Answer from the drawing. Dimensions are ordinates in mm from the lowest x, y and z of the part. Give positions to 0.01 mm unless a question says otherwise; leave off trailing zeros. Order: outer loops, then holes, each group sorted by start corner. A loop starts at its lowest first (then second) coordinate and runs counter-clockwise, first axis right, second up.
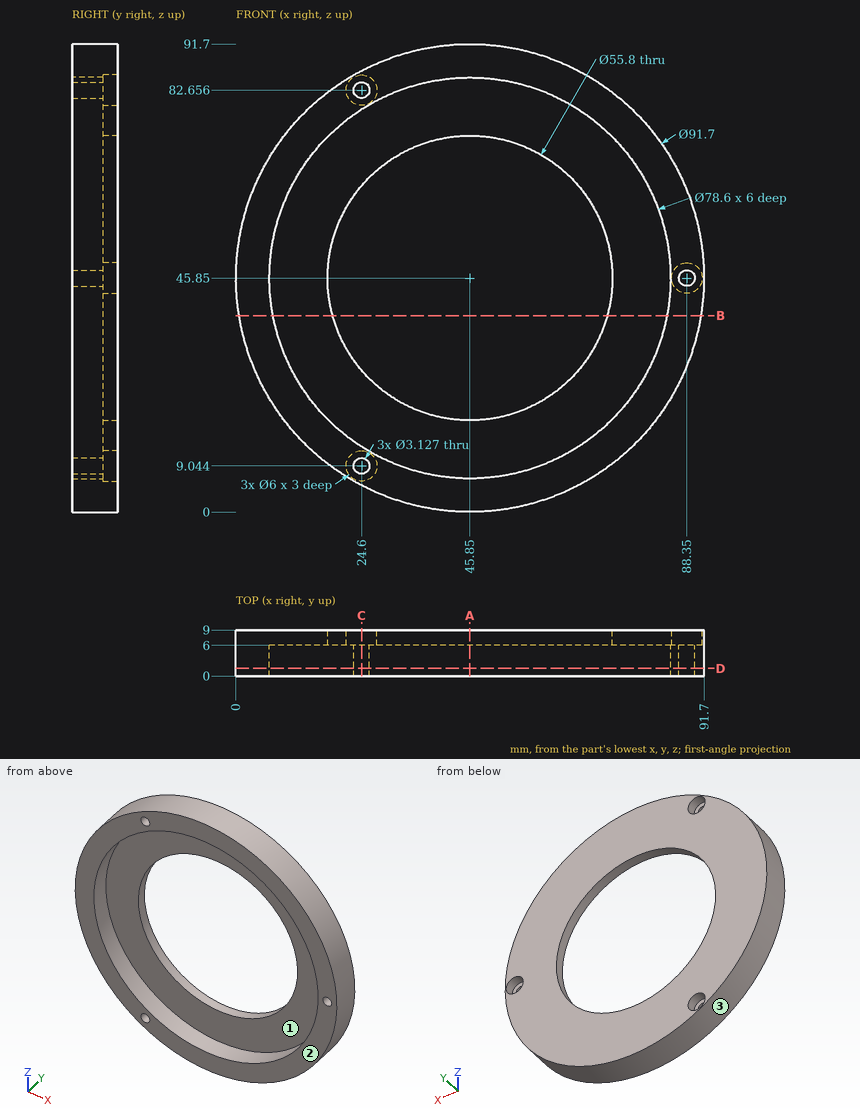
1) For a pull along Z with two mould halves and no side action, classify the marked faces 1, 2 and 3 as released by +Z, released by -Z, zero draft, split by the parting line, or undercut.
Final values:
face 1: undercut
face 2: zero draft
face 3: split by the parting line
2) The part is cut by section D-D on y = 1.5. Determine the outline of the cut face in (x, z).
Final values:
outline: circle Ø91.7 at (45.85, 45.85); hole circle Ø78.6 at (45.85, 45.85); hole circle Ø3.13 at (24.6, 9.04); hole circle Ø3.13 at (24.6, 82.66); hole circle Ø3.13 at (88.35, 45.85)
3) Given pin 1 (5 mm diameter, centred on x = 35.5, z = 18.5, fed in from -Y); pin 2 (4 mm diameter, centred on x = 40, y = 5.5, fed in from -Z); pin 3 (5 mm diameter, centred on y = 2.5, z = 66, fed in from -X), each flat-ended and moving along its own axis, determine where each tip first touches the part or whether it passes through.
Final values:
pin 1: stops at y = 6
pin 2: stops at z = 0.16
pin 3: stops at x = 3.53
4) Consider L1, parallel to X at y = 2.95, z = 45.85; L2, parallel to X at y = 6.85, z = 45.85; L3, parallel to X at y = 7.5, z = 35. Determine where each line is inside the solid, lowest interval first.
Final values:
L1: x = 0 to 6.55, 85.15 to 86.79, 89.91 to 91.7
L2: x = 0 to 17.95, 73.75 to 85.35, 91.35 to 91.7
L3: x = 1.3 to 20.15, 71.55 to 90.4
5) The part is cut by section A-A on x = 45.85. Determine the outline of the cut face in (y, z).
Final values:
outline: (0, 0) - (9, 0) - (9, 17.95) - (6, 17.95) - (6, 6.55) - (0, 6.55) - close; (0, 85.15) - (6, 85.15) - (6, 73.75) - (9, 73.75) - (9, 91.7) - (0, 91.7) - close
6) The part is cut by section C-C on x = 24.6. Determine the outline of the cut face in (y, z).
Final values:
outline: (0, 5.22) - (9, 5.22) - (9, 6.04) - (6, 6.04) - (6, 7.48) - (0, 7.48) - close; (0, 10.61) - (6, 10.61) - (6, 12.04) - (9, 12.04) - (9, 27.77) - (6, 27.77) - (6, 12.79) - (0, 12.79) - close; (0, 78.91) - (6, 78.91) - (6, 63.93) - (9, 63.93) - (9, 79.66) - (6, 79.66) - (6, 81.09) - (0, 81.09) - close; (0, 84.22) - (6, 84.22) - (6, 85.66) - (9, 85.66) - (9, 86.48) - (0, 86.48) - close
7) The part is cut by section B-B on z = 38.5. Determine the outline of the cut face in (x, y), and give its area (3 significant figures).
Final values:
outline: (0.59, 0) - (7.24, 0) - (7.24, 6) - (18.94, 6) - (18.94, 9) - (0.59, 9) - close; (72.76, 6) - (84.46, 6) - (84.46, 0) - (91.11, 0) - (91.11, 9) - (72.76, 9) - close
area: 190 mm2
